Geometry check sheet. Reference: the model listing, model coordinates, mm. A direction names the side the tool comes from. Give positions to 0.01 mm unless a question says otherwise; leave off trailing zeros. Write each loop counter-clockwise with the first axis right and the second up, starting at its lowest first coordinate (ties: lowest second). Pieces come first, ordered by that corner, then holes. Notation, with made-up numbers: M 19,87.25 L 59,87.25 A14 cw 59,103.25 Z; hole C 68.5,-38.75 d1. An arc over 180 degrees is marked long. One line per item, written item: value. Start each with the question number.
1. Scan lines: line 1 (X direction, y = 1, z = 53); line 2 (X direction, y = 64, z = 8.5); line 3 (Y direction, x = 0, z = 21). Record each from-to range of solid material in increasing order.
2. Cross-section at B-B on x = 44. Record the cut outline in (y, z), then the cut area to 3 significant figures.
3. Tool access check on faces 4 (the face through (-7.5, 12, 38)), 5 (the face through (19, 72, 25)), 6 (the face through (-19, 72, 25)), 7 (the face through (7.5, 12, 38)). Record the directions out of +Z, -Z, +X, -X, +Y, -Y that give a thin tool (end or side, any length) a straight path to the whole face; none if there is none.
4. Release check for a two-part mould opening along X. For faces 1 (the face through (35.077, 0.091, 54.172)), 2 (the face through (-63, 5, 21)), 3 (the face through (35, 6.5, 45)) record: pulls with the +X half, pulls with the -X half, needs draft (parallel to the pull), parting line crosses it, or undercut.
5. Gauge pin test, flat ends, axial feed: pin 1 (2 mm diameter, centred on x = 19, y = 59, fed in from +Z); pin 2 (7 mm diameter, centred on y = 70, z = 29.5, fed in from -X); pin 3 (5 mm diameter, centred on y = 22.5, z = 26.5, fed in from -X). Record the tip position at first contact, or that the pin passes through.
6. Cross-section at D-D on z = 53. Count the separate pieces of the cut face and the enclosed holes in it, then the cut area to 3 significant figures.
7. Cross-section at C-C on x = 26.5. Record the cut outline in (y, z).
8. Cross-section at A-A on y = 44.5. Record the cut outline in (x, z), then the cut area to 3 significant figures.
from build123d import *

# Parameters (mm, degrees)
SKETCH1_W           = 126
SKETCH1_H           = 13
BOSS_EXTRUDE1_DEPTH = 78
SKETCH1_3_R         = 9
BOSS_EXTRUDE2_DEPTH = 13
SKETCH1_4_R         = 25
SKETCH1_4_R_2       = 16
BOSS_EXTRUDE3_DEPTH = 51
BOSS_EXTRUDE4_DEPTH = 38
SKETCH2_R           = 9
CUT_EXTRUDE1_DEPTH  = 127.419935137
FILLET1_R           = 25


with BuildPart() as part:
    # Sketch1 → Boss-Extrude1 (new body)
    with BuildSketch(Plane.XY):
        Rectangle(SKETCH1_W, SKETCH1_H)
    extrude(amount=BOSS_EXTRUDE1_DEPTH)

    # Sketch1<3> → Boss-Extrude2 (add)
    with BuildSketch(Plane.XY):
        with BuildLine():
            Line((-63, 83.5), (-63, 6.5))
            Line((-63, 6.5), (63, 6.5))
            Line((63, 6.5), (63, 83.5))
            Line((63, 83.5), (19, 83.5))
            Line((19, 83.5), (19, 60.748076809))
            ThreePointArc((19, 60.748076809), (23.452078799, 53.160254038), (25, 44.5))
            ThreePointArc((25, 44.5), (-8.660254038, 21.047921201), (-19, 60.748076809))
            Line((-19, 60.748076809), (-19, 83.5))
            Line((-19, 83.5), (-63, 83.5))
        make_face()
        with Locations(Location((-44, 58.5, 0), (0, 0, 180))):
            Circle(SKETCH1_3_R, mode=Mode.SUBTRACT)
        with Locations(Location((44, 58.5, 0), (0, 0, 180))):
            Circle(SKETCH1_3_R, mode=Mode.SUBTRACT)
    extrude(amount=BOSS_EXTRUDE2_DEPTH)

    # Sketch1<4> → Boss-Extrude3 (add)
    with BuildSketch(Plane.XY):
        with Locations(Location((0, 44.5, 0), (0, 0, 139.464197889))):
            Circle(SKETCH1_4_R)
        with Locations((0, 44.5)):
            Circle(SKETCH1_4_R_2, mode=Mode.SUBTRACT)
    extrude(amount=BOSS_EXTRUDE3_DEPTH)

    # Sketch1<5> → Boss-Extrude4 (add)
    with BuildSketch(Plane.XY):
        with BuildLine():
            Line((-9, 83.5), (-19, 83.5))
            Line((-19, 83.5), (-19, 60.748076809))
            ThreePointArc((-19, 60.748076809), (0, 69.5), (19, 60.748076809))
            Line((19, 60.748076809), (19, 83.5))
            Line((19, 83.5), (9, 83.5))
            ThreePointArc((9, 83.5), (0, 74.5), (-9, 83.5))
        make_face()
    extrude(amount=BOSS_EXTRUDE4_DEPTH)

    # Sketch2 → Cut-Extrude1 (cut, through all)
    with BuildSketch(Plane(origin=(0, 6.5, 0), x_dir=(1, 0, 0), z_dir=(0, 1, 0))):
        with Locations(Location((-44, -53, 0), (0, 0, 270))):
            Circle(SKETCH2_R)
        with Locations(Location((44, -53, 0), (0, 0, 90))):
            Circle(SKETCH2_R)
    extrude(amount=-CUT_EXTRUDE1_DEPTH, mode=Mode.SUBTRACT)

    # Fillet1
    fillet1_edges = [part.edges().sort_by_distance(p)[0] for p in [
        (-63, 83.5, 6.5),
        (63, 83.5, 6.5),
    ]]
    fillet(fillet1_edges, radius=FILLET1_R)

    # Sketch4 → Loft4 section 0
    with BuildSketch(Plane(origin=(-7.5, 0, 0), x_dir=(0, 0, -1), z_dir=(1, 0, 0))):
        with BuildLine():
            Line((-78, 6.5), (-51, 20.651519965))
            Line((-51, 20.651519965), (-13, 20.651519965))
            Line((-13, 20.651519965), (-13, 6.5))
            Line((-13, 6.5), (-78, 6.5))
        make_face()
    # Sketch6 → Loft4 section 1
    with BuildSketch(Plane(origin=(0, 0, 0), x_dir=(0, 0, -1), z_dir=(1, 0, 0))):
        with BuildLine():
            Line((-78, 6.5), (-51, 19.5))
            Line((-51, 19.5), (-13, 19.5))
            Line((-13, 19.5), (-13, 6.5))
            Line((-13, 6.5), (-78, 6.5))
        make_face()
    # Sketch5 → Loft4 section 2
    with BuildSketch(Plane(origin=(7.5, 0, 0), x_dir=(0, 0, -1), z_dir=(1, 0, 0))):
        with BuildLine():
            Line((-78, 6.5), (-51, 20.651519965))
            Line((-51, 20.651519965), (-13, 20.651519965))
            Line((-13, 20.651519965), (-13, 6.5))
            Line((-13, 6.5), (-78, 6.5))
        make_face()
    loft()


solid = part.part
Report:
1. line 1: x = -63 to -53, -35 to 35, 53 to 63
1. line 2: x = -62.39 to -51.12, -36.88 to 36.88, 51.12 to 62.39
1. line 3: y = -6.5 to 28.5, 60.5 to 74.5
2. outline: M -6.5,0 L 49.5,0 L 49.5,13 L 6.5,13 L 6.5,44 L -6.5,44 Z; M -6.5,62 L 6.5,62 L 6.5,78 L -6.5,78 Z; M 67.5,0 L 82.77,0 L 82.77,13 L 67.5,13 Z
2. area: 1,540 mm^2
3. face 4: +Z, -X
3. face 5: +Z, +X, +Y
3. face 6: +Z, -X, +Y
3. face 7: +Z, +X
4. face 1: undercut
4. face 2: pulls with the -X half
4. face 3: needs draft
5. pin 1: stops at z = 51
5. pin 2: stops at x = -19
5. pin 3: stops at x = -15.64
6. separate pieces: 3
6. enclosed holes: 0
6. area: 1,360 mm^2
7. outline: M -6.5,0 L 83.5,0 L 83.5,13 L 6.5,13 L 6.5,78 L -6.5,78 Z
8. outline: M -63,0 L -16,0 L -16,51 L -25,51 L -25,13 L -63,13 Z; M 16,0 L 63,0 L 63,13 L 25,13 L 25,51 L 16,51 Z
8. area: 1,910 mm^2
